Could you check a few things on this model? Use its own coordinates, in mm. Face numbers are marked on the shaded views. A direction names the side the tool comes from. Coordinates: 2 decimals unless noted, no trailing zeros. Write each loop counter-clockwise with the first axis right and the second up, starting at its lowest first coordinate (ties: lowest second). Pieces come first, ordered by that corner, then holes. Notation, with made-up numbers: M -28.5,-31.75 L -15.5,-31.75 A19 ccw -15.5,4.25 Z; hole C -31.75,8.5 d1. An arc over 180 degrees is marked long. Answer as CSV lines item,"result". Start each with the question number.
Item 1: Suppose I cut it at D-D, the plane z = -13.5. Write out the boundary of the cut face in (x, y), and give its area (3 significant figures).
Item 2: On a 3-axis mill with a long thin cutter (end or side, diameter ignored), from which of +Z, -Z, +X, -X, +Y, -Y can I reach the whole of each face in a straight line? I mean the marked faces 5, 6, 7 and 8. Say none if no direction works.
Item 3: If I drill on line 1 along Y through (x, z) = (9.5, -43.5); line 2 along Y through (x, z) = (8, 4); line 3 along Z through (x, y) = (3.5, 18), over which ranges is the centre line in solid material (lowest first)? Write a range as [from, to].
Item 4: Suppose I cut it at C-C, the plane y = 35.5. Write out the boundary of the cut face in (x, z), and give its area (3 significant figures).
Item 5: Suppose I cut it at A-A, the plane z = -38.15. Write out the boundary of the cut face in (x, y), and give its area (3 significant figures).
Item 6: Suppose I cut it at B-B, the plane x = 1.9. Write out the boundary of the cut face in (y, z).
Item 7: We'd pull the mould along Y, two halves only. Please class the marked faces 1, 2, 3 and 4: +Y half, -Y half, draft (parallel to the pull), parting line (faces both ways), or undercut.
Item 8: I'm going to push flat-ended pins straight in: P1, Ø1.1, axis at x = 8.5, z = -40.5, coming from the +Y side; P2, Ø3, axis at x = 10, z = -42.5, coming from the +Y side; P3, Ø1, axis at x = 8.5, y = 36.5, coming from the +Z side; P4, Ø8, axis at x = 13.5, z = -12.5, coming from the -Y side. Where does each tip first touch, or does it pass through?
```python
from build123d import *

# Parameters (mm, degrees)
BOSS_EXTRU_1_DEPTH      = 20.2
ESQUISSE2_R             = 4.10078125
ESQUISSE2_R_2           = 2.375
ENL_V_MAT_EXTRU_1_DEPTH = 62.192646617
ESQUISSE3_R             = 2.95
BOSS_EXTRU_2_DEPTH      = 5.7
ESQUISSE4_R             = 1.8
BOSS_EXTRU_3_DEPTH      = 3.3
ESQUISSE5_R             = 6.6
BOSS_EXTRU_4_DEPTH      = 1.5
ESQUISSE6_W             = 7.5
ESQUISSE6_H             = 5
BOSS_EXTRU_5_DEPTH      = 1
BOSS_EXTRU_6_DEPTH      = 4


with BuildPart() as part:
    # Esquisse1 → Boss.-Extru.1 (new body)
    with BuildSketch(Plane(origin=(0, 0, 0), x_dir=(0, 0, -1), z_dir=(1, 0, 0))):
        Polygon((0, 0), (40.2, 0), (40.2, 27.6), (49.3, 27.6), (49.3, 30.1), (40.2, 30.1), (40.2, 38.5), (0, 38.5), (0, 30.1), (-9.1, 30.1), (-9.1, 27.6), (0, 27.6), align=None)
    extrude(amount=BOSS_EXTRU_1_DEPTH)

    # Esquisse2 → Enlèv. mat.-Extru.1 (cut, through all)
    with BuildSketch(Plane(origin=(0, 30.1, 0), x_dir=(1, 0, 0), z_dir=(0, 1, 0))):
        with Locations((10.1, 51.80078125)):
            Circle(ESQUISSE2_R)
        with Locations(Location((5.475, 45.075, 0), (0, 0, 270))):
            Circle(ESQUISSE2_R_2)
        with Locations(Location((14.725, 45.075, 0), (0, 0, 270))):
            Circle(ESQUISSE2_R_2)
        with Locations(Location((14.725, -4.875, 0), (0, 0, 270))):
            Circle(ESQUISSE2_R_2)
        with Locations(Location((5.475, -4.875, 0), (0, 0, 270))):
            Circle(ESQUISSE2_R_2)
        with Locations((10.1, -11.60078125)):
            Circle(ESQUISSE2_R)
    extrude(amount=-ENL_V_MAT_EXTRU_1_DEPTH, mode=Mode.SUBTRACT)

    # Esquisse3 → Boss.-Extru.2 (add)
    with BuildSketch(Plane(origin=(0, 38.5, 0), x_dir=(1, 0, 0), z_dir=(0, 1, 0))):
        with Locations(Location((10.1, 29.95, 0), (0, 0, 90))):
            Circle(ESQUISSE3_R)
    extrude(amount=BOSS_EXTRU_2_DEPTH)

    # Esquisse4 → Boss.-Extru.3 (add)
    with BuildSketch(Plane(origin=(0, 38.5, 0), x_dir=(1, 0, 0), z_dir=(0, 1, 0))):
        with Locations(Location((1.9, 29.95, 0), (0, 0, 90))):
            Circle(ESQUISSE4_R)
        with Locations(Location((10.1, 38.15, 0), (0, 0, 90))):
            Circle(ESQUISSE4_R)
        with Locations(Location((18.3, 29.95, 0), (0, 0, 90))):
            Circle(ESQUISSE4_R)
        with Locations(Location((10.1, 21.75, 0), (0, 0, 90))):
            Circle(ESQUISSE4_R)
    extrude(amount=BOSS_EXTRU_3_DEPTH)

    # Esquisse5 → Boss.-Extru.4 (add)
    with BuildSketch(Plane(origin=(0, 38.5, 0), x_dir=(1, 0, 0), z_dir=(0, 1, 0))):
        with Locations((10.1, 29.95)):
            Circle(ESQUISSE5_R)
    extrude(amount=BOSS_EXTRU_4_DEPTH)

    # Esquisse6 → Boss.-Extru.5 (add)
    with BuildSketch(Plane(origin=(0, 0, -40.2), x_dir=(-1, 0, 0), z_dir=(0, 0, -1))):
        with Locations((-10.1, 5)):
            Rectangle(ESQUISSE6_W, ESQUISSE6_H)
    extrude(amount=BOSS_EXTRU_5_DEPTH)

    # Esquisse7 → Boss.-Extru.6 (add)
    with BuildSketch(Plane(origin=(0, 0, -41.2), x_dir=(-1, 0, 0), z_dir=(0, 0, -1))):
        with BuildLine():
            Line((-11.5, 6.5), (-8.7, 6.5))
            ThreePointArc((-8.7, 6.5), (-7.2, 5), (-8.7, 3.5))
            Line((-8.7, 3.5), (-11.5, 3.5))
            ThreePointArc((-11.5, 3.5), (-13, 5), (-11.5, 6.5))
        make_face()
    extrude(amount=BOSS_EXTRU_6_DEPTH)


solid = part.part
```
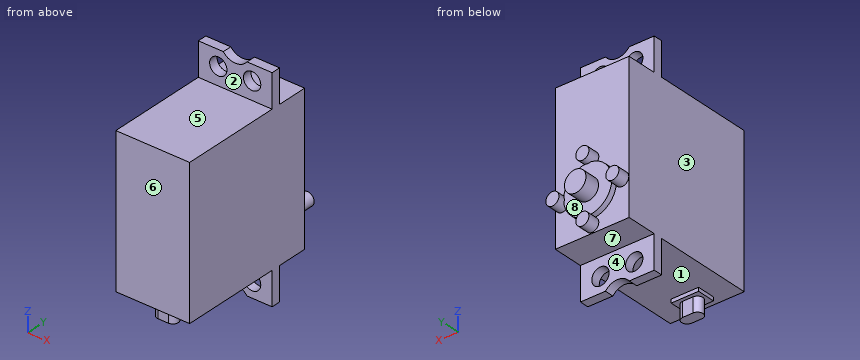
Ans:
1,outline,"M 0,0 L 20.2,0 L 20.2,38.5 L 0,38.5 Z"
1,area,"778 mm^2"
2,face 5,"+Z, +X, -X, -Y"
2,face 6,"+Z, -Z, +X, -X, -Y"
2,face 7,"-Z, +X, -X, +Y"
2,face 8,"+Y"
3,line 1,"y = [3.5, 6.5], [27.6, 30.1]"
3,line 2,"y = [27.6, 30.1]"
3,line 3,"z = [-40.2, 0]"
4,outline,"M 0,-40.2 L 20.2,-40.2 L 20.2,0 L 0,0 Z"
4,area,"812 mm^2"
5,outline,"M 0,0 L 20.2,0 L 20.2,38.5 L 11.9,38.5 L 11.9,41.8 L 8.3,41.8 L 8.3,38.5 L 0,38.5 Z"
5,area,"790 mm^2"
6,outline,"M 0,-40.2 L 27.6,-40.2 L 27.6,-49.3 L 30.1,-49.3 L 30.1,-40.2 L 38.5,-40.2 L 38.5,-31.75 L 41.8,-31.75 L 41.8,-28.15 L 38.5,-28.15 L 38.5,0 L 30.1,0 L 30.1,9.1 L 27.6,9.1 L 27.6,0 L 0,0 Z"
7,face 1,"undercut"
7,face 2,"-Y half"
7,face 3,"draft"
7,face 4,"+Y half"
8,P1,"stops at y = 38.5"
8,P2,"stops at y = 30.1"
8,P3,"stops at z = 0"
8,P4,"stops at y = 0"
